Can you work these out from the model? Positions are in its coordinate system, mm. Give positions to 0.01 mm unless a question says otherwise; leave off trailing zeros. Order: outer loops, then holes, each group sorted by start corner. A loop starts at its lowest first (then second) coordinate and runs counter-clockwise, first axis right, second up.
Item 1: If I drill on line 1 along Y through (x, z) = (51.5, 2.85); line 2 along Y through (x, z) = (111, 1.8); line 3 along X through (y, z) = (27.5, 1.15), over which ranges is the centre line in solid material (lowest first)?
Item 2: I want a section at D-D, the plane y = 31. Write out the boundary of the cut face in (x, z).
Item 3: I want a section at C-C, the plane x = 28. Write out the boundary of the cut face in (y, z).
Item 4: I'm going to push flat-ended pins straight in: pin 1 Ø1.5 at (y, z) = (19.5, 1.5) entering from +X; pin 2 Ø0.9 at (y, z) = (50, 1) entering from +X; pin 3 Ø1 at (x, z) = (44, 1.5) entering from -Y. Where does each tip first touch, or does it pass through?
Item 5: I want a section at A-A, the plane x = 58. Write out the boundary of the cut face in (y, z), then the cut area to 3 significant figures.
Item 6: I want a section at B-B, the plane z = 1.35. Write out the boundary of the cut face in (x, y), then the cut area to 3 significant figures.
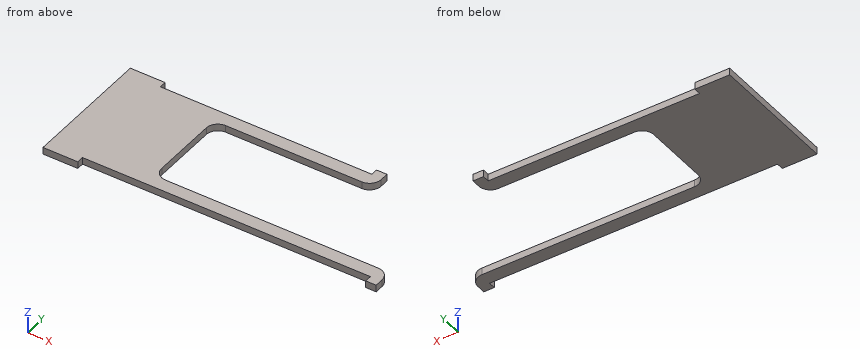
Autodesk Inventor part; units mm, degrees
ref_plane "YZ Plane" through (0, 0, 0) normal (1, 0, 0) x (0, 1, 0)
ref_plane "XZ Plane" through (0, 0, 0) normal (0, 1, 0) x (-1, 0, 0)
ref_plane "XY Plane" through (0, 0, 0) normal (0, 0, 1) x (1, 0, 0)
sketch "Эскиз3" plane through (0, 0, 0) normal (0, 0, 1) x (1, 0, 0)
  line L0 (106.2, 49.8) -> (15, 49.8)
  line L1 (0, 49.8) -> (0, 0)
  line L2 (0, 0) -> (0, -3)
  line L3 (0, -3) -> (15, -3)
  line L4 (15, -3) -> (15, 0)
  line L5 (0, 49.8) -> (0, 52.8)
  line L6 (0, 52.8) -> (15, 52.8)
  line L7 (15, 52.8) -> (15, 49.8)
  line L8 (138.7, 5.7) -> (47, 5.7)
  line L9 (42, 10.7) -> (42, 39.1)
  line L10 (47, 44.1) -> (105.7, 44.1)
  line L11 (110.7, 49.1) -> (110.7, 52.8)
  line L12 (110.7, 52.8) -> (106.2, 52.8)
  line L13 (106.2, 52.8) -> (106.2, 49.8)
  arc A0 (105.7, 44.1) -> (110.7, 49.1) centre (105.7, 49.1) ccw
  arc A1 (42, 10.7) -> (47, 5.7) centre (47, 10.7) ccw
  arc A2 (47, 44.1) -> (42, 39.1) centre (47, 39.1) ccw
  line L14 (15, 0) -> (139.2, 0)
  line L15 (139.2, 0) -> (139.2, -3)
  line L16 (139.2, -3) -> (143.7, -3)
  line L17 (143.7, -3) -> (143.7, 0.7)
  arc A3 (143.7, 0.7) -> (138.7, 5.7) centre (138.7, 0.7) ccw
  point P0 (42, 5.7)
  point P1 (42, 44.1)
  point P2 (110.7, 44.1)
  point P3 (143.7, 5.7)
  dimension "d10" = 15
  dimension "d12" = 42
  dimension "d13" = 4.5
  dimension "d14" = 5
  dimension "d15" = 5.7
  dimension "d16" = 5
  dimension "d17" = 91.2
  dimension "d18" = 3
  dimension "d20" = 5
  dimension "d21" = 124.2
  dimension "d22" = 49.8
extrude "Выдавливание3" add sketch "Эскиз3" along normal blind 3
equation "\"d6\" = thickness_steel"
equation "\"tolerance_plazma\" = 0.1"
equation "\"thickness_steel\" = 3"
equation "\"d_main_screw_holes\" = 6.1"
equation "\"thickness_profile_tibea\" = 3"
equation "\"hight_shaft_shift\" = 37"
equation "\"thickness_profile_femur\" = 3"
equation "\"width_shaft_shift\" = 35"
equation "\"width_flattened_surface\" = 12"
properties part number "femur_reinforcement_tibea_steel" material "Сталь"
Results list:
1. line 1: y = 0 to 5.7, 44.1 to 49.8
1. line 2: y = 0 to 5.7
1. line 3: x = 0 to 42
2. outline: (0, 0) - (42, 0) - (42, 3) - (0, 3) - close
3. outline: (0, 0) - (49.8, 0) - (49.8, 3) - (0, 3) - close
4. pin 1: stops at x = 42
4. pin 2: stops at x = 110.7
4. pin 3: stops at y = 0
5. outline: (0, 0) - (5.7, 0) - (5.7, 3) - (0, 3) - close; (44.1, 0) - (49.8, 0) - (49.8, 3) - (44.1, 3) - close
5. area: 34.2 mm2
6. outline: (0, -3) - (15, -3) - (15, 0) - (139.2, 0) - (139.2, -3) - (143.7, -3) - (143.7, 0.7) arc R5 ccw to (138.7, 5.7) - (47, 5.7) arc R5 cw to (42, 10.7) - (42, 39.1) arc R5 cw to (47, 44.1) - (105.7, 44.1) arc R5 ccw to (110.7, 49.1) - (110.7, 52.8) - (106.2, 52.8) - (106.2, 49.8) - (15, 49.8) - (15, 52.8) - (0, 52.8) - close
6. area: 3,180 mm2
